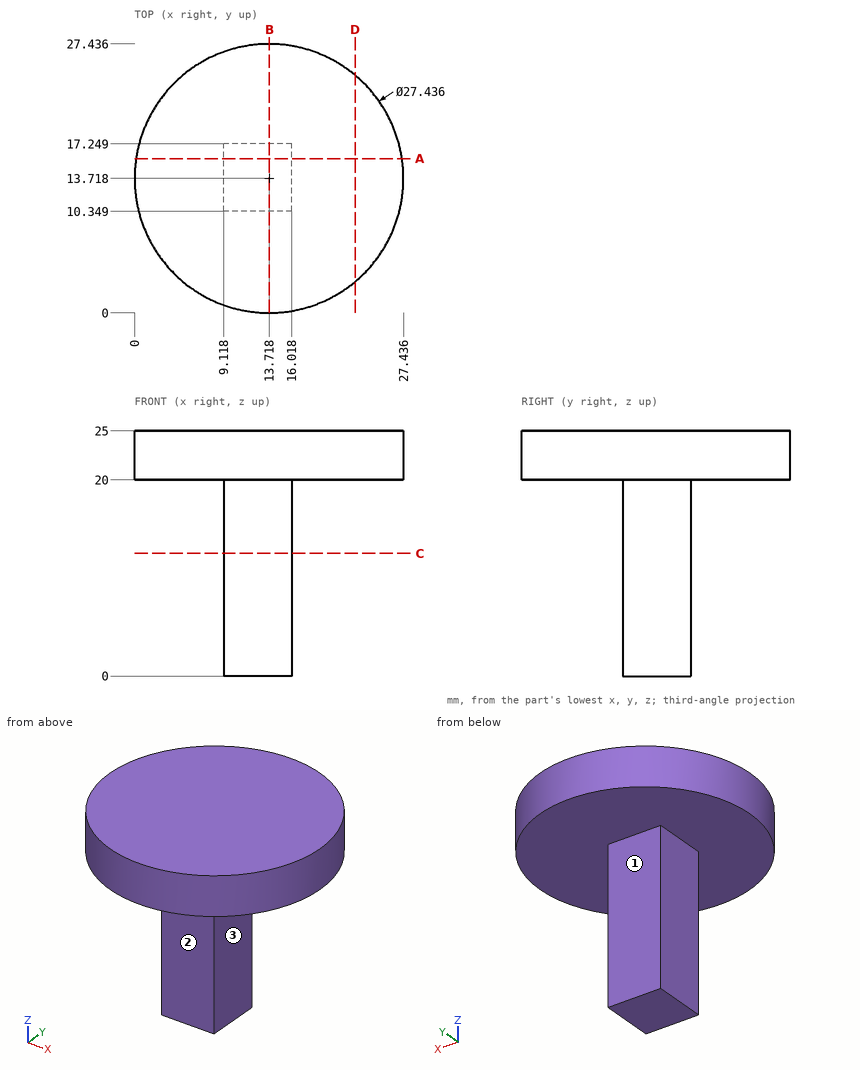
The drawing under review shows one solid part. Ordinate dimensions are in mm from its lowest x, y, z. A direction names the side the tool comes from. Round coordinates to 2 decimals unless told otherwise and drop trailing zeros. Write each loop counter-clockwise with the first axis right and the second up, starting at its lowest first coordinate (ties: lowest second). Pieces come first, ordered by that corner, then holes. Notation, with made-up numbers: (72, -38) -> (111, -38) arc R28 ccw to (111, -17) -> close; hole circle Ø9 at (24, 42.25). An arc over 180 degrees is marked (long way). Put each result on its own line as item: value.
Q1. Machinability: for the marked faces 1, 2 and 3, which of the approach directions +Z, -Z, +X, -X, +Y, -Y give a long, thin tool a straight path to every point of the face, cutting with its end or side? Answer none if there is none.
Determined:
face 1: -Z, +X, -X, +Y
face 2: -Z, +X, -X, -Y
face 3: -Z, +X, +Y, -Y
Q2. Consider section C-C on z = 12.5. State the section outline as (x, y) points, and give its area (3 significant figures).
Determined:
outline: (9.12, 10.35) -> (16.02, 10.35) -> (16.02, 17.25) -> (9.12, 17.25) -> close
area: 47.6 mm^2
Q3. Consider section A-A on y = 15.75. State the section outline as (x, z) points (1 decimal), and give its area (3 significant figures).
Determined:
outline: (0.2, 20) -> (9.1, 20) -> (9.1, 0) -> (16, 0) -> (16, 20) -> (27.3, 20) -> (27.3, 25) -> (0.2, 25) -> close
area: 274 mm^2
Q4. Consider section B-B on x = 13.75. State the section outline as (y, z) points, and give its area (3 significant figures).
Determined:
outline: (0, 20) -> (10.35, 20) -> (10.35, 0) -> (17.25, 0) -> (17.25, 20) -> (27.44, 20) -> (27.44, 25) -> (0, 25) -> close
area: 275 mm^2
Q5. To check wall thickness, follow L1, parallel to Z at x = 8, y = 4.25; L2, parallel to X at y = 13.25, z = 3.5; L3, parallel to Y at x = 14.5, z = 12.5. State the ranges of each line that lie inside material, in increasing order. Write a range as [from, to].
Determined:
L1: z = [20, 25]
L2: x = [9.12, 16.02]
L3: y = [10.35, 17.25]
Q6. Clearance check with flat-ended pins moving along their axes: pin 1 Ø7.5 at (y, z) = (14.5, 8) entering from -X; pin 2 Ø1 at (x, y) = (11.5, 3) entering from -Z; pin 3 Ø5.5 at (x, z) = (11, 13.5) entering from -Y. State where each tip first meets the part, or that it passes through.
Determined:
pin 1: stops at x = 9.12
pin 2: stops at z = 20
pin 3: stops at y = 10.35
Q7. Consider section D-D on x = 22.5. State the section outline as (y, z) points, and give its area (3 significant figures).
Determined:
outline: (3.18, 20) -> (24.26, 20) -> (24.26, 25) -> (3.18, 25) -> close
area: 105 mm^2
